Design review of the part built by this model. Coordinates are the model's own, in mm. A direction names the side the tool comes from. Round coordinates to 2 decimals unless told otherwise and drop trailing zeros. Write each loop counter-clockwise with the first axis right and the second up, starting at its lowest first coordinate (ties: lowest second). Pieces come first, ordered by that corner, then holes. Notation, with made-up numbers: M 61,41.5 L 76,41.5 A28 ccw 76,65.5 Z; hole C 12,29 d1. An arc over 180 degrees is marked long. Use CSV: the item, a comma, the result in double quotes.
from build123d import *

# Parameters (mm, degrees)
F0_R     = 25.4
F0_R_2   = 6.35
F1_DEPTH = 25.4


with BuildPart() as f1:
    # F0 (on Top) → F1 (new body)
    with BuildSketch(Plane.XY):
        Circle(F0_R)
        with BuildLine():
            Line((-17.78, 0), (17.78, 0))
            ThreePointArc((17.78, 0), (0, -17.78), (-17.78, 0))
        make_face(mode=Mode.SUBTRACT)
        with Locations((-10.795, 12.7)):
            Circle(F0_R_2, mode=Mode.SUBTRACT)
        with Locations((10.795, 12.7)):
            Circle(F0_R_2, mode=Mode.SUBTRACT)
    extrude(amount=F1_DEPTH)


solid = f1.part
1) Wall thickness on line 1 along X through (y, z) = (14, 5.75); line 2 along Y through (x, z) = (-16, 17.5); line 3 along Y through (x, z) = (11, 20.5): over which ranges is each line inside the solid? List them lowest first. Write a range as [from, to].
Answers:
line 1,"[-21.19, -17.01], [-4.58, 4.58], [17.01, 21.19]"
line 2,"[-19.73, -7.75], [0, 9.06], [16.34, 19.73]"
line 3,"[-22.89, -13.97], [0, 6.35], [19.05, 22.89]"
2) Add section D-D on x = 6. Write out the cut boundary in (y, z), then the cut area to 3 significant figures.
Answers:
outline,"M -24.68,0 L -16.74,0 L -16.74,25.4 L -24.68,25.4 Z; M 0,0 L 8.54,0 L 8.54,25.4 L 0,25.4 Z; M 16.86,0 L 24.68,0 L 24.68,25.4 L 16.86,25.4 Z"
area,"617 mm²"
3) The part is to be moulded in two halves that separate along X. For faces 3 (the face through (-0.4, 0.4, 0)), 4 (the face through (-15.475, 16.992, 12.522)), 5 (the face through (0.391, -17.776, 12.522)), 6 (the face through (-5.506, -24.796, 12.522)), say which applies: released by +X, released by -X, zero draft, split by the parting line, or undercut.
Answers:
face 3,"zero draft"
face 4,"undercut"
face 5,"undercut"
face 6,"split by the parting line"
4) For pin 1 Ø3 at (x, z) = (-8.5, 3.5) entering from -Y; pin 2 Ø6 at (x, z) = (17, 18) entering from -Y; pin 3 Ø8 at (y, z) = (4.5, 7) entering from +X, all flat-tipped, find the tip position at first contact; note any pin that passes through.
Answers:
pin 1,"y = -24.42"
pin 2,"y = -21.19"
pin 3,"x = 25.4"
5) Add section B-B on y = 18. Write out the cut boundary in (x, z), then the cut area to 3 significant figures.
Answers:
outline,"M -17.92,0 L -14.29,0 L -14.29,25.4 L -17.92,25.4 Z; M -7.3,0 L 7.3,0 L 7.3,25.4 L -7.3,25.4 Z; M 14.29,0 L 17.92,0 L 17.92,25.4 L 14.29,25.4 Z"
area,"555 mm²"
6) Machinability: for faces 1 (the face through (-0.4, 0.4, 25.4)), 2 (the face through (0, 0, 13)), which of the approach directions +Z, -Z, +X, -X, +Y, -Y give a long, thin tool a straight path to every point of the face, cutting with its end or side? Answer none if there is none.
Answers:
face 1,"+Z, +X, -X, +Y, -Y"
face 2,"+Z, -Z"
7) Add section A-A on x = 0. Write out the cut boundary in (y, z), then the cut area to 3 significant figures.
Answers:
outline,"M -25.4,0 L -17.78,0 L -17.78,25.4 L -25.4,25.4 Z; M 0,0 L 25.4,0 L 25.4,25.4 L 0,25.4 Z"
area,"839 mm²"
8) Add section C-C on z = 17.75. Write out the cut boundary in (x, y) (3 decimals).
Answers:
outline,"C 0,0 d50.8; hole M -17.78,0 A17.78 ccw 17.78,0 Z; hole C -10.795,12.7 d12.7; hole C 10.795,12.7 d12.7"
